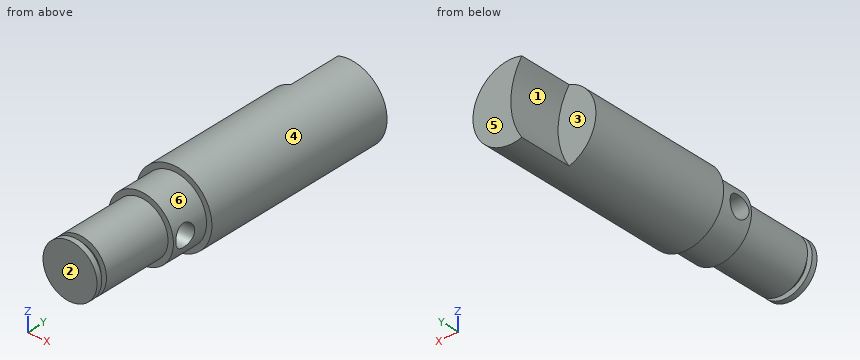
```python
from build123d import *

# Parameters (mm, degrees)
SKETCH1_R               = 2.5
BOSS_EXTRUDE1_DEPTH     = 0.5
SKETCH2_R               = 2
BOSS_EXTRUDE2_DEPTH     = 0.5
SKETCH3_R               = 2.5
BOSS_EXTRUDE3_DEPTH     = 6.5
SKETCH4_R               = 3
BOSS_EXTRUDE4_DEPTH     = 3.5
SKETCH5_R               = 3.5
BOSS_EXTRUDE5_DEPTH     = 18.5
CUT_EXTRUDE2_START      = 24.5
CUT_EXTRUDE2_DEPTH      = 5
CUT_EXTRUDE3_DEPTH      = 30.912372022
CUT_EXTRUDE3_DEPTH_BACK = 30.912372022
SKETCH10_R              = 1


with BuildPart() as part:
    # Sketch1 → Boss-Extrude1 (new body)
    with BuildSketch(Plane(origin=(0, 0, 0), x_dir=(1, 0, 0), z_dir=(0, 1, 0))):
        with Locations(Location((0, 0, 0), (0, 0, 270))):
            Circle(SKETCH1_R)
    extrude(amount=BOSS_EXTRUDE1_DEPTH)

    # Sketch2 → Boss-Extrude2 (add)
    with BuildSketch(Plane(origin=(0, 0.5, 0), x_dir=(1, 0, 0), z_dir=(0, 1, 0))):
        with Locations(Location((0, 0, 0), (0, 0, 270))):
            Circle(SKETCH2_R)
    extrude(amount=BOSS_EXTRUDE2_DEPTH)

    # Sketch3 → Boss-Extrude3 (add)
    with BuildSketch(Plane(origin=(0, 1, 0), x_dir=(1, 0, 0), z_dir=(0, 1, 0))):
        with Locations(Location((0, 0, 0), (0, 0, 270))):
            Circle(SKETCH3_R)
    extrude(amount=BOSS_EXTRUDE3_DEPTH)

    # Sketch4 → Boss-Extrude4 (add)
    with BuildSketch(Plane(origin=(0, 7.5, 0), x_dir=(1, 0, 0), z_dir=(0, 1, 0))):
        with Locations(Location((0, 0, 0), (0, 0, 270))):
            Circle(SKETCH4_R)
    extrude(amount=BOSS_EXTRUDE4_DEPTH)

    # Sketch5 → Boss-Extrude5 (add)
    with BuildSketch(Plane(origin=(0, 11, 0), x_dir=(1, 0, 0), z_dir=(0, 1, 0))):
        with Locations(Location((0, 0, 0), (0, 0, 270))):
            Circle(SKETCH5_R)
    extrude(amount=BOSS_EXTRUDE5_DEPTH)

    # Sketch8 → Cut-Extrude2 (cut)
    with BuildSketch(Plane(origin=(0, 0, 0), x_dir=(1, 0, 0), z_dir=(0, 1, 0)).offset(CUT_EXTRUDE2_START)):
        with BuildLine():
            ThreePointArc((-1.020833333, 3.347820083), (0, 0), (-1.020833333, -3.347820083))
            ThreePointArc((-1.020833333, -3.347820083), (-3.5, 0), (-1.020833333, 3.347820083))
        make_face()
    extrude(amount=CUT_EXTRUDE2_DEPTH, mode=Mode.SUBTRACT)

    # Sketch10 → Cut-Extrude3 (cut, two sides: drawn at the far end of the back side and taken through both)
    with BuildSketch(Plane(origin=(0, 0, 0), x_dir=(0, 0, -1), z_dir=(1, 0, 0)).offset(-CUT_EXTRUDE3_DEPTH_BACK)):
        with Locations((0, 8.75)):
            Circle(SKETCH10_R)
    extrude(amount=CUT_EXTRUDE3_DEPTH + CUT_EXTRUDE3_DEPTH_BACK, mode=Mode.SUBTRACT)


solid = part.part
```
Could you check a few things on this model? Use its own coordinates, in mm. Face numbers are marked on the shaded views. A direction names the side the tool comes from. Coordinates: 2 decimals unless noted, no trailing zeros. Loops run counter-clockwise (first coordinate to the right, second up) from the corner with the lowest first, then second, coordinate; pieces in that order, holes last. Notation, with made-up numbers: M 57,-27 L 70,-27 A23 ccw 70,-1 Z; hole C 32,-40 d11. An arc over 180 degrees is marked long. Put each result on its own line as item: value. Start each with the question number.
(1) Thinking about a two-plate mould opening in Z: for the marked faces 1, 2, 3 and 4, which applies, pulls with the +Z half, pulls with the -Z half, needs draft (parallel to the pull), parting line crosses it, or undercut?
(2) Will these pins go through, and if not, where does the flat tip stop? P1, Ø2, axis at x = -2, y = 19, coming from the +Z side; P2, Ø4, axis at x = -1.5, y = 22.5, coming from the +Z side; P3, Ø1.8, axis at y = 8.75, z = 0, coming from the +X side; P4, Ø1.5, axis at x = -1, z = 0.5, coming from the +Y side.
(3) For the marked faces 5 and 6, which set-ups out of +Z, -Z, +X, -X, +Y, -Y let a thin tool reach every point of the face, with its end or its side?
(4) Suppose I cut it at A-A on z = 0. Please give me the cut outline in (x, y).
(5) Suppose I cut it at B-B on y = 8.75. Please give me the cut outline in (x, z).
(6) Suppose I cut it at D-D on x = 0.5. Please give me the cut outline in (y, z).
(7) I need wall thicknesses on line 1 (Y direction, x = 1.5, z = 0); line 2 (Y direction, x = 1, z = 2.25); line 3 (Z direction, x = -1, y = 16). Which ranges of each line are inside material? Lowest first, please. Write a range as from..to.
(8) Suppose I cut it at C-C on z = -1.5. Please give me the cut outline in (x, y).
Solutions:
1. face 1: undercut
1. face 2: needs draft
1. face 3: undercut
1. face 4: parting line crosses it
2. P1: stops at z = 3.35
2. P2: stops at z = 3.5
2. P3: passes through
2. P4: stops at y = 24.5
3. face 5: +Z, -Z, +X, -X, +Y
3. face 6: -Y
4. outline: M -3.5,11 L -3,11 L -3,9.75 L 3,9.75 L 3,11 L 3.5,11 L 3.5,29.5 L 0,29.5 L 0,24.5 L -3.5,24.5 Z; M -3,7.5 L -2.5,7.5 L -2.5,1 L -2,1 L -2,0.5 L -2.5,0.5 L -2.5,0 L 2.5,0 L 2.5,0.5 L 2,0.5 L 2,1 L 2.5,1 L 2.5,7.5 L 3,7.5 L 3,7.75 L -3,7.75 Z
5. outline: M -2.83,-1 A3 ccw 2.83,-1 Z; M -2.83,1 L 2.83,1 A3 ccw Z
6. outline: M 0,-2.45 L 0.5,-2.45 L 0.5,-1.94 L 1,-1.94 L 1,-2.45 L 7.5,-2.45 L 7.5,-2.96 L 11,-2.96 L 11,-3.46 L 29.5,-3.46 L 29.5,3.46 L 11,3.46 L 11,2.96 L 7.5,2.96 L 7.5,2.45 L 1,2.45 L 1,1.94 L 0.5,1.94 L 0.5,2.45 L 0,2.45 Z; hole C 8.75,0 d2
7. line 1: y = 0..7.75, 9.75..29.5
7. line 2: y = 0..0.5, 1..29.5
7. line 3: z = -3.35..3.35
8. outline: M -3.16,11 L -2.6,11 L -2.6,7.5 L -2,7.5 L -2,1 L -1.32,1 L -1.32,0.5 L -2,0.5 L -2,0 L 2,0 L 2,0.5 L 1.32,0.5 L 1.32,1 L 2,1 L 2,7.5 L 2.6,7.5 L 2.6,11 L 3.16,11 L 3.16,29.5 L -0.19,29.5 L -0.19,24.5 L -3.16,24.5 Z
